```python
from build123d import *

# Parameters (mm, degrees)
F5_DEPTH = 120
F9_DEPTH = 5


with BuildPart() as f5:
    # F4 (on Top) → F5 (new body, through all)
    with BuildSketch(Plane.XY):
        Polygon((17.6776695297, 17.6776695297), (0, 25), (-17.6776695297, 17.6776695297), (-25, 0), (-17.6776695297, -17.6776695297), (0, -25), (17.6776695297, -17.6776695297), (25, 0), align=None)
    extrude(amount=F5_DEPTH)

    # F6 (on offset) → F8 section 0
    with BuildSketch(Plane.XY.offset(120)):
        Polygon((21.2132034356, 21.2132034356), (0, 30), (-21.2132034356, 21.2132034356), (-30, 0), (-21.2132034356, -21.2132034356), (0, -30), (21.2132034356, -21.2132034356), (30, 0), align=None)
    # F7 (on offset) → F8 section 1
    with BuildSketch(Plane.XY.offset(155)):
        Polygon((29.4525549142, 29.4525549142), (0, 41.6522026062), (-29.4525549142, 29.4525549142), (-41.6522026062, 0), (-29.4525549142, -29.4525549142), (0, -41.6522026062), (29.4525549142, -29.4525549142), (41.6522026062, 0), align=None)
    loft()

    # F9 (add, through all): a face of the model
    f9_faces = [f5.faces().sort_by_distance(p)[0] for p in [
        (0, 0, 155),
    ]]
    extrude(f9_faces, amount=F9_DEPTH)

    # F9_face (on face) → F11 section 0
    with BuildSketch(Plane.XY.offset(160), mode=Mode.PRIVATE) as f11_s0:
        Polygon((29.4525549142, -29.4525549142), (41.6522026062, 0), (29.4525549142, 29.4525549142), (0, 41.6522026062), (-29.4525549142, 29.4525549142), (-41.6522026062, 0), (-29.4525549142, -29.4525549142), (0, -41.6522026062), align=None)
    loft([f11_s0.sketch, Vertex(0, 0, 170)])


solid = f5.part
```
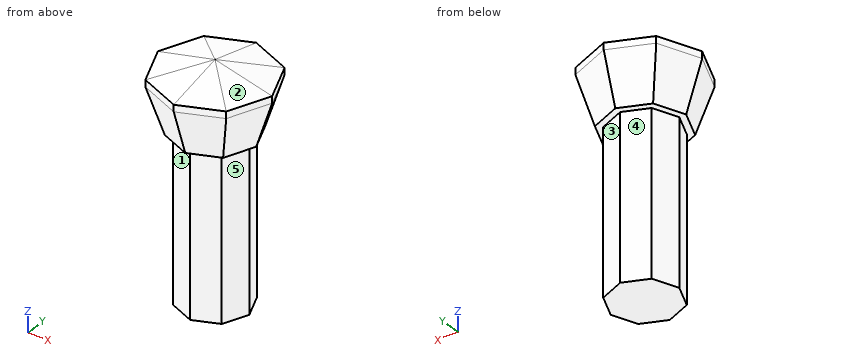
Model file for the job. Use its own axes, mm. Face numbers are marked on the shaded views. A direction names the side the tool comes from. Coordinates: 2 decimals unless noted, no trailing zeros. Loops run counter-clockwise (first coordinate to the right, second up) from the corner with the lowest first, then second, coordinate; pieces in that order, holes last. Notation, with made-up numbers: (-12.5, 47.25) - (38.5, 47.25) arc R30 ccw to (38.5, 71.25) - close; hole circle Ø2 at (29.25, -30.5). An arc over 180 degrees is marked (long way). Answer as a JSON object with one key per item and string values. Group by question number.
(1) Probe line 1 along X through (y, z) = (18, 94.5); line 2 along Z through (x, y) = (19, -11.5); line 3 along X through (y, z) = (-11, 67.5). List the from-to ranges inside material, lowest first.
(2) Tool access for the marked faces 1, 2, 3, 4 and 5: list every direction of +Z, -Z, +X, -X, +Y, -Y with a clear straight run to the whole face (end or side of a thin tool).
(3) Cut at A-A (z = 85). Give the cut face in (x, y), then the cut area to 3 significant figures.
(4) Flat gauge pins, fed straight in: pin 1 (12 mm diameter, centred on y = 15.5, z = 134.5, fed in from -X); pin 2 (6 mm diameter, centred on x = 9.5, z = 121.5, fed in from -Y); pin 3 (12 mm diameter, centred on y = -17, z = 63.5, fed in from +X); pin 4 (18 mm diameter, centred on x = 4, y = -8, fed in from -Z). Where does each tip first touch, or does it go through?
Geometry says:
{
 "1": {"line 1": "x = -16.9 to 16.9", "line 2": "z = 0 to 164.29", "line 3": "x = -20.44 to 20.44"},
 "2": {"face 1": "-Z, -X, -Y", "face 2": "+Z, +X, -Y", "face 3": "-Z, +X, +Y", "face 4": "-Z, -X, +Y", "face 5": "-Z, +X, -Y"},
 "3": {"outline": "(-25, 0) - (-17.68, -17.68) - (0, -25) - (17.68, -17.68) - (25, 0) - (17.68, 17.68) - (0, 25) - (-17.68, 17.68) - close", "area": "1,770 mm^2"},
 "4": {"pin 1": "stops at x = -31.6", "pin 2": "stops at y = -28.16", "pin 3": "stops at x = 20.44", "pin 4": "stops at z = 0"}
}
